Source: CAD feature listing. Evaluate the final solid. Frame: model axes, mm. Give positions to 0.01 mm unless a question says otherwise; leave off trailing zeros. Order: outer loops, then holes, each group sorted by start corner. A loop starts at its lowest first (then second) coordinate and runs counter-clockwise, first axis right, second up. Notation, with made-up numbers: (75.25, 4) - (97.25, 4) arc R6 cw to (97.25, 14) - close; hole circle Ø5 at (39.5, -5). An arc over 180 degrees is marked (long way). One line per item, written item: value. Start each with the question number.
Autodesk Inventor part; units mm, degrees
ref_plane "YZ Plane" through (0, 0, 0) normal (1, 0, 0) x (0, 1, 0)
ref_plane "XZ Plane" through (0, 0, 0) normal (0, 1, 0) x (-1, 0, 0)
ref_plane "XY Plane" through (0, 0, 0) normal (0, 0, 1) x (1, 0, 0)
sketch "Эскиз1" plane through (0, 0, 0) normal (0, 0, 1) x (1, 0, 0)
  line L0 (-3.7707, 0) -> (-3.7707, 1.5)
  line L1 (-3.7707, 1.5) -> (3.7293, 1.5)
  line L2 (3.7293, 1.5) -> (3.7293, 0)
  line L3 (3.7293, 0) -> (-3.7707, 0)
  point P0 (0, 0)
  dimension "d0" = 1.5
  dimension "d1" = 7.5
revolve "Вращение1" add sketch "Эскиз1" angle 360 about axis through (3.7293, 0, 0) along (-1, 0, 0)
sketch "Эскиз4" plane through (0, 0, 0) normal (0, 0, 1) x (1, 0, 0)
  line L0 (3.7293, 1.5) -> (3.7293, -1.5)
  line L1 (3.7293, 0) -> (16.0293, 0)
  line L2 (16.2293, -0.2) -> (16.2293, -12.5)
  arc A0 (16.2293, -0.2) -> (16.0293, 0) centre (16.0293, -0.2) ccw
  point P0 (0, 0)
  point P1 (16.2293, 0)
  dimension "d3" = 12.5
  dimension "d4" = 12.5
  dimension "d5" = 0.2
ref_plane "РабПлоскость1" through (3.7293, 0, 0) normal (1, 0, 0) x (0, 0, -1)
sketch "Эскиз5" plane through (3.7293, 0, 0) normal (1, 0, 0) x (0, 0, -1)
  circle A0 centre (0, 0) radius 0.25
  dimension "d7" = 0.5
sweep "Сдвиг1" add profiles "Эскиз5" path "Эскиз4" path curves L1 A0 L2
mirror "Зеркальное отражение1" about plane through (0, 0, 0) normal (1, 0, 0) of "Сдвиг1"
properties part number "КС147А"
1. Section B-B on y = -4.5. Return the cut outline in (x, z), then the cut area to 3 significant figures.
2. Section A-A on x = -7. Return the cut outline in (y, z).
3. Ray query, L1, parallel to X at y = -7.75, z = 0; L2, parallel to Z at x = -7, y = 0; L3, parallel to X at y = 0.5, z = 0.85. Return the intervals inside material, ascending.
4. Contact query for a flat-ended pin moving along its axis: pin 1 Ø1.5 at (y, z) = (0.5, 0.5) entering from +X. Output: stop coordinate, or through.
Data:
1. outline: circle Ø0.5 at (-16.23, 0); circle Ø0.5 at (16.23, 0)
1. area: 0.393 mm2
2. outline: circle Ø0.5 at (0, 0)
3. L1: x = -16.48 to -15.98, 15.98 to 16.48
3. L2: z = -0.25 to 0.25
3. L3: x = -3.77 to 3.73
4. pin 1: stops at x = 16.46
